from build123d import *

# Parameters (mm, degrees)
SKETCH1_R           = 5
BOSS_EXTRUDE1_DEPTH = 10.5
SKETCH2_R           = 3
CUT_EXTRUDE1_DEPTH  = 6
FILLET1_R           = 1
CHAMFER1_SIZE       = 0.5
CHAMFER1_SIZE2      = 1.37373871


with BuildPart() as part:
    # Sketch1 → Boss-Extrude1 (new body)
    with BuildSketch(Plane(origin=(0, 0, 0), x_dir=(1, 0, 0), z_dir=(0, 1, 0))):
        Circle(SKETCH1_R)
    extrude(amount=BOSS_EXTRUDE1_DEPTH)

    # Sketch2 → Cut-Extrude1 (cut)
    with BuildSketch(Plane.XZ):
        Circle(SKETCH2_R)
    extrude(amount=-CUT_EXTRUDE1_DEPTH, mode=Mode.SUBTRACT)

    # Fillet1
    fillet1_edges = [part.edges().sort_by_distance(p)[0] for p in [
        (-5, 10.5, 0),
    ]]
    fillet(fillet1_edges, radius=FILLET1_R)

    # Chamfer1
    chamfer1_edges = [part.edges().sort_by_distance(p)[0] for p in [
        (-5, 0, 0),
    ]]
    chamfer1_side = [part.faces().sort_by_distance(p)[0] for p in [
        (-4.858578644, 0, 0),
    ]]
    chamfer(chamfer1_edges, length=CHAMFER1_SIZE, length2=CHAMFER1_SIZE2, reference=chamfer1_side[0])


solid = part.part
Input: part model. Units: mm. Frame: model coordinates. A direction names the side the tool comes from. Give positions to 0.01 mm unless a question says otherwise; leave off trailing zeros. Order: outer loops, then holes, each group sorted by start corner. A loop starts at its lowest first (then second) coordinate and runs counter-clockwise, first axis right, second up. Notation, with made-up numbers: (11, 87) - (57, 87) arc R12 cw to (57, 94) - close; hole circle Ø2 at (77.25, 21.5). An arc over 180 degrees is marked (long way). Write each question's results on one line, items separated by ' | '.
Item 1: Material intervals for line 1 along Z through (x, y) = (0, 2.3); line 2 along Z through (x, y) = (-4, 5); line 3 along Y through (x, z) = (-2.5, 1.25), sorted ascending.
A:
line 1: z = -5 to -3, 3 to 5 | line 2: z = -3 to 3 | line 3: y = 6 to 10.5
Item 2: Contact query for flat-ended pins moving along their axis: pin 1 Ø3 at (x, z) = (0, -0.5) entering from -Y; pin 2 Ø2 at (y, z) = (1.5, 2.5) entering from +X; pin 3 Ø2 at (y, z) = (4.5, 2) entering from +X. Output: stop coordinate, or through.
A:
pin 1: stops at y = 6 | pin 2: stops at x = 4.77 | pin 3: stops at x = 4.9
Item 3: Draft query along Z for faces 3 (the cylindrical face through (-1.08, 5.38, 4.88)), 4 (the flat face through (0, 10.5, 0)), 5 (the cylindrical face through (-3, 3, 0)). Return one class per face: released by +Z, released by -Z, zero draft, split by the parting line, or undercut.
A:
face 3: split by the parting line | face 4: zero draft | face 5: undercut
Item 4: Section C-C (y = 6.25). Return loops of the section in (x, z).
A:
outline: circle Ø10 at (0, 0)
Item 5: Access query for faces 1 (the flat face through (1, 0, 3)), 2 (the flat face through (0, 6, 0)). Directions: +Z, -Z, +X, -X, +Y, -Y. A direction counts if a zero-diameter tool reaches every point of the face in a straight line with its end or side. Return the directions, or none.
A:
face 1: +Z, -Z, +X, -X, -Y | face 2: -Y
Item 6: Section B-B (z = 0). Return loops of the section in (x, y), and give its area (3 significant figures).
A:
outline: (-5, 1.37) - (-4.5, 0) - (-3, 0) - (-3, 6) - (3, 6) - (3, 0) - (4.5, 0) - (5, 1.37) - (5, 9.5) arc R1 ccw to (4, 10.5) - (-4, 10.5) arc R1 ccw to (-5, 9.5) - close | area: 67.9 mm^2
Item 7: Section D-D (y = 3.75). Return loops of the section in (x, z).
A:
outline: circle Ø10 at (0, 0); hole circle Ø6 at (0, 0)
Item 8: Section A-A (x = 0). Return loops of the section in (y, z), and give its area (3 significant figures).
A:
outline: (0, -4.5) - (1.37, -5) - (9.5, -5) arc R1 ccw to (10.5, -4) - (10.5, 4) arc R1 ccw to (9.5, 5) - (1.37, 5) - (0, 4.5) - (0, 3) - (6, 3) - (6, -3) - (0, -3) - close | area: 67.9 mm^2
